Check sheet for the drawn part. Datum: minimum x, y, z corner. Units: mm. Coordinates: 2 decimals unless noted, no trailing zeros. Write each loop counter-clockwise with the first axis right and the second up, starting at its lowest first coordinate (ties: lowest second). Pieces come first, ordered by that corner, then holes. Notation, with made-up numbers: (74.5, 61) -> (112.5, 61) arc R18 ccw to (112.5, 73) -> close; hole circle Ø11 at (88.25, 50). An arc over 180 degrees is marked (long way). Write each question's results on one line, items separated by ' | '. Start each with the question number.
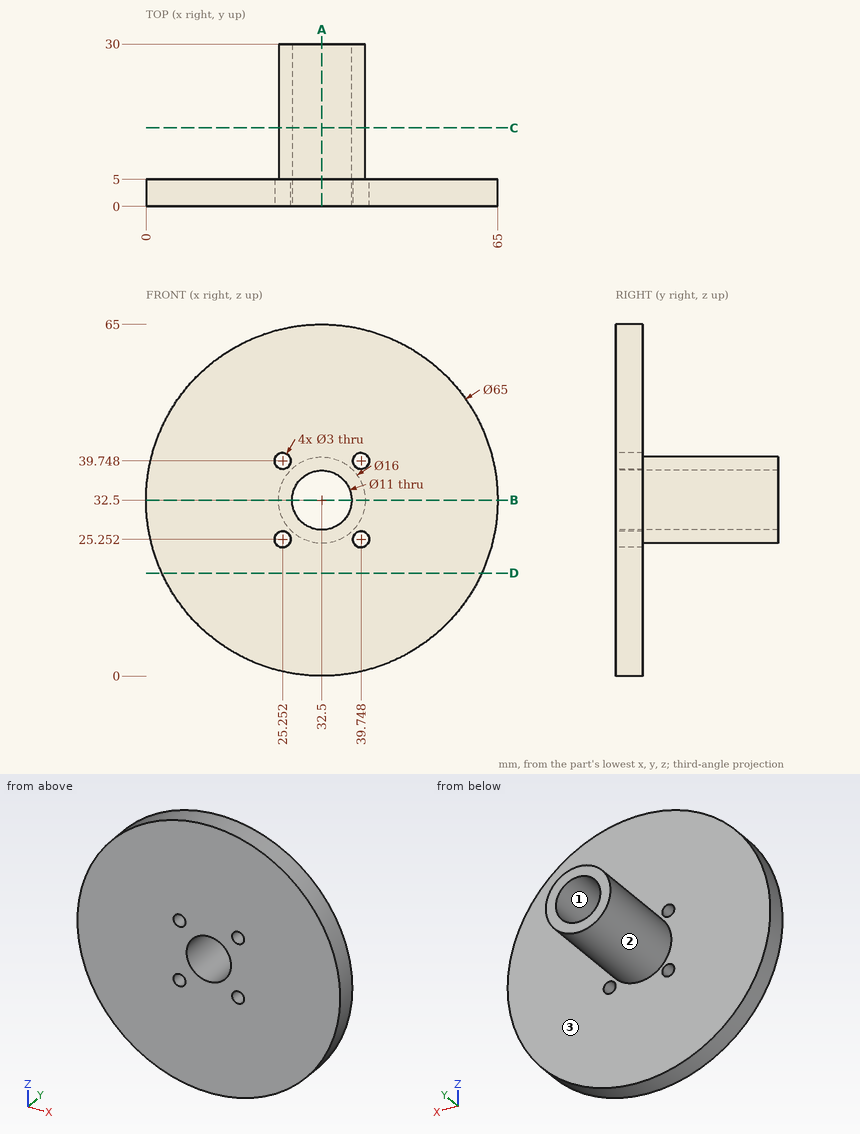
1. Sectioned sample at C-C on y = 14.5. Record the cut outline in (x, z).
2. Mould release check, pull along Z, two halves, no side actions. Record for the marked faces 1, 2 and 3: +Z half, -Z half, draft (parallel to the pull), parting line (faces both ways), or undercut.
3. Depth check by flat-ended pin: pin 1 Ø6 at (x, y) = (18.5, 8.5) entering from +Z; pin 2 Ø10 at (y, z) = (25, 43.5) entering from +X; pin 3 Ø1.5 at (x, y) = (30.5, 19.5) entering from -Z; pin 4 Ø4 at (y, z) = (5, 11.5) entering from +X. Enter the tip coordinate at first touch or a pass-through.
4. Sectioned sample at A-A on x = 32.5. Record the cut outline in (y, z), plus the area to 3 significant figures.
5. Sectioned sample at D-D on z = 19. Record the cut outline in (x, y).
6. Sectioned sample at B-B on z = 32.5. Record the cut outline in (x, y), plus the area to 3 significant figures.
7. Material ranges on probe 1 along Z at (x, y) = (32.5, 15); probe 2 along Y at (x, z) = (49.5, 58), recorded low to high. Write a range as from..to.
Computed values:
1) outline: circle Ø16 at (32.5, 32.5); hole circle Ø11 at (32.5, 32.5)
2) face 1: undercut | face 2: parting line | face 3: draft
3) pin 1: passes through | pin 2: stops at x = 37.79 | pin 3: stops at z = 24.6 | pin 4: stops at x = 58.87
4) outline: (0, 0) -> (5, 0) -> (5, 24.5) -> (30, 24.5) -> (30, 27) -> (0, 27) -> close; (0, 38) -> (30, 38) -> (30, 40.5) -> (5, 40.5) -> (5, 65) -> (0, 65) -> close | area: 395 mm^2
5) outline: (2.94, 0) -> (62.06, 0) -> (62.06, 5) -> (2.94, 5) -> close
6) outline: (0, 0) -> (27, 0) -> (27, 30) -> (24.5, 30) -> (24.5, 5) -> (0, 5) -> close; (38, 0) -> (65, 0) -> (65, 5) -> (40.5, 5) -> (40.5, 30) -> (38, 30) -> close | area: 395 mm^2
7) probe 1: z = 24.5..27, 38..40.5 | probe 2: y = 0..5
